Can you work these out from the model? Positions are in its coordinate system, mm. Give positions to 0.01 mm unless a question says otherwise; leave off trailing zeros. Loops run counter-clockwise (first coordinate to the right, second up) from the corner with the lowest first, then second, coordinate; pieces in that order, holes last.
from build123d import *

# Parameters (mm, degrees)
SKETCH1_R           = 11.2
BOSS_EXTRUDE1_DEPTH = 3.175


with BuildPart() as part:
    # Sketch1 → Boss-Extrude1 (new body)
    with BuildSketch(Plane.XY):
        with BuildLine():
            Line((-139.7, -203.2), (139.7, -203.2))
            ThreePointArc((139.7, -203.2), (157.660512242, -195.760512242), (165.1, -177.8))
            Line((165.1, -177.8), (165.1, 177.8))
            ThreePointArc((165.1, 177.8), (157.660512242, 195.760512242), (139.7, 203.2))
            Line((139.7, 203.2), (-139.7, 203.2))
            ThreePointArc((-139.7, 203.2), (-157.660512242, 195.760512242), (-165.1, 177.8))
            Line((-165.1, 177.8), (-165.1, -177.8))
            ThreePointArc((-165.1, -177.8), (-157.660512242, -195.760512242), (-139.7, -203.2))
        make_face()
        with Locations((-139.7, 76.2)):
            Circle(SKETCH1_R, mode=Mode.SUBTRACT)
        with Locations((139.7, 76.2)):
            Circle(SKETCH1_R, mode=Mode.SUBTRACT)
        with BuildLine():
            Line((-101.6, -152.4), (101.6, -152.4))
            ThreePointArc((101.6, -152.4), (110.580256121, -148.680256121), (114.3, -139.7))
            Line((114.3, -139.7), (114.3, -50.8))
            ThreePointArc((114.3, -50.8), (110.580256121, -41.819743879), (101.6, -38.1))
            Line((101.6, -38.1), (-101.6, -38.1))
            ThreePointArc((-101.6, -38.1), (-110.580256121, -41.819743879), (-114.3, -50.8))
            Line((-114.3, -50.8), (-114.3, -139.7))
            ThreePointArc((-114.3, -139.7), (-110.580256121, -148.680256121), (-101.6, -152.4))
        make_face(mode=Mode.SUBTRACT)
        with BuildLine():
            Line((-101.6, -12.7), (101.6, -12.7))
            ThreePointArc((101.6, -12.7), (110.580256121, -8.980256121), (114.3, 0))
            Line((114.3, 0), (114.3, 38.1))
            ThreePointArc((114.3, 38.1), (110.580256121, 47.080256121), (101.6, 50.8))
            Line((101.6, 50.8), (-101.6, 50.8))
            ThreePointArc((-101.6, 50.8), (-110.580256121, 47.080256121), (-114.3, 38.1))
            Line((-114.3, 38.1), (-114.3, 0))
            ThreePointArc((-114.3, 0), (-110.580256121, -8.980256121), (-101.6, -12.7))
        make_face(mode=Mode.SUBTRACT)
        with BuildLine():
            Line((-101.6, 152.4), (101.6, 152.4))
            ThreePointArc((101.6, 152.4), (110.580256121, 148.680256121), (114.3, 139.7))
            Line((114.3, 139.7), (114.3, 88.9))
            ThreePointArc((114.3, 88.9), (110.580256121, 79.919743879), (101.6, 76.2))
            Line((101.6, 76.2), (-101.6, 76.2))
            ThreePointArc((-101.6, 76.2), (-110.580256121, 79.919743879), (-114.3, 88.9))
            Line((-114.3, 88.9), (-114.3, 139.7))
            ThreePointArc((-114.3, 139.7), (-110.580256121, 148.680256121), (-101.6, 152.4))
        make_face(mode=Mode.SUBTRACT)
    extrude(amount=BOSS_EXTRUDE1_DEPTH)


solid = part.part
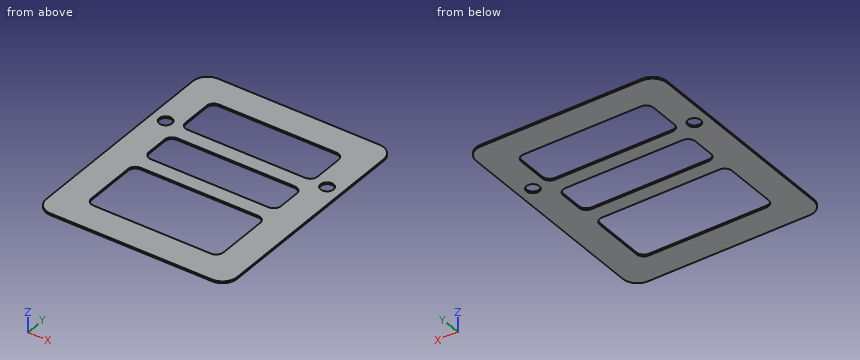
(1) Please list where these lines run through material, in increasing order: probe 1 along Y at (x, z) = (-101, 0.8); probe 2 along Y at (x, z) = (-139.7, 1.85); probe 3 along X at (y, z) = (-116.5, 2.15).
Returned:
probe 1: y = -203.2 to -152.4, -38.1 to -12.7, 50.8 to 76.2, 152.4 to 203.2
probe 2: y = -203.2 to 65, 87.4 to 203.2
probe 3: x = -165.1 to -114.3, 114.3 to 165.1
(2) Suppose I cut it at A-A on x = 40. List the corners of the cut face in (y, z) for me (3 decimals).
Returned:
outline: (-203.2, 0) - (-152.4, 0) - (-152.4, 3.175) - (-203.2, 3.175) - close; (-38.1, 0) - (-12.7, 0) - (-12.7, 3.175) - (-38.1, 3.175) - close; (50.8, 0) - (76.2, 0) - (76.2, 3.175) - (50.8, 3.175) - close; (152.4, 0) - (203.2, 0) - (203.2, 3.175) - (152.4, 3.175) - close
(3) Suppose I cut it at C-C on x = 135.5. List the corners of the cut face in (y, z) for me (3 decimals).
Returned:
outline: (-203.2, 0) - (65.817, 0) - (65.817, 3.175) - (-203.2, 3.175) - close; (86.583, 0) - (203.2, 0) - (203.2, 3.175) - (86.583, 3.175) - close
(4) Suppose I cut it at B-B on y = -72. List the corners of the cut face in (x, z) for me (3 decimals), plus the area to 3 significant figures.
Returned:
outline: (-165.1, 0) - (-114.3, 0) - (-114.3, 3.175) - (-165.1, 3.175) - close; (114.3, 0) - (165.1, 0) - (165.1, 3.175) - (114.3, 3.175) - close
area: 323 mm2
(5) Suppose I cut it at D-D on z = 2.2. Give the number of separate pieces and of enclosed holes in the cut face, plus the area to 3 significant figures.
Returned:
separate pieces: 1
enclosed holes: 5
area: 75,200 mm2
